Autodesk Inventor part; units mm, degrees
ref_plane "YZ Plane" through (0, 0, 0) normal (1, 0, 0) x (0, 1, 0)
ref_plane "XZ Plane" through (0, 0, 0) normal (0, 1, 0) x (-1, 0, 0)
ref_plane "XY Plane" through (0, 0, 0) normal (0, 0, 1) x (1, 0, 0)
sketch "Sketch1" plane through (0, 0, 0) normal (0, 1, 0) x (-1, 0, 0)
  circle A0 centre (0, 0) radius 20
  dimension "d0" = 40
extrude "Extrusion1" add sketch "Sketch1" along normal blind 26
sketch "Sketch2" plane through (0, 26, 0) normal (0, 1, 0) x (1, 0, 0)
  circle A0 centre (0, 0) radius 19.95
  dimension "d3" = 39.9
extrude "Extrusion2" add sketch "Sketch2" along normal blind 5
sketch "Sketch3" plane through (0, 31, 0) normal (0, 1, 0) x (1, 0, 0)
  circle A0 centre (0, 0) radius 10
  dimension "d6" = 20
extrude "Extrusion3" add sketch "Sketch3" along normal blind 5
sketch "Sketch4" plane through (0, 36, 0) normal (0, 1, 0) x (1, 0, 0)
  circle A0 centre (0, 0) radius 3
  dimension "d9" = 6
extrude "Extrusion4" add sketch "Sketch4" along normal blind 15
sketch "Sketch5" plane through (0, 51, 0) normal (0, 1, 0) x (1, 0, 0)
  circle A0 centre (0, 0) radius 3
  circle A1 centre (0, 0) radius 3
  line L0 (-1.9261, -2.3) -> (1.9261, -2.3)
  dimension "d12" = 2.3
extrude "Extrusion5" cut sketch "Sketch5" against normal blind 10 contours L0 A0 picked at (0.4482, -2.4273)
fillet "Fillet1" radius 2 1 edges at (20, 0, 0)
chamfer "Chamfer1" distance 1 angle 45 2 edges at (-19.95, 31, 0) (-10, 36, 0)
chamfer "Chamfer2" distance 0.5 angle 45 2 edges at (2.7183, 51, 1.2692) (-1.2692, 51, -2.7183)
sketch "Sketch6" plane through (0, 31, 0) normal (0, 1, 0) x (1, 0, 0)
  point P0 (0, 0)
  point P1 (0, 15)
  point P2 (-12.9904, -7.5)
  point P3 (12.9904, -7.5)
  dimension "d23" = 15
  dimension "d26" = 360
hole "Hole1" at (0, 31, -15) at (-12.9904, 31, 7.5) at (12.9904, 31, 7.5) direction (0, -1, 0) diameter 3.4 depth 5 tip angle 118 countersink diameter 3.8 countersink angle 90
properties part number "Encoder" material "Stainless Steel"
Build history of the part. All positions in model axes, mm. A direction names the side the tool comes from. Give positions to 0.01 mm unless a question says otherwise; leave off trailing zeros. Write each loop counter-clockwise with the first axis right and the second up, starting at its lowest first coordinate (ties: lowest second). Pieces come first, ordered by that corner, then holes. Notation, with made-up numbers: (0.5, -6.75) - (22.5, -6.75) arc R25 cw to (22.5, 7.25) - close; hole circle Ø6 at (85, 12.5). An arc over 180 degrees is marked (long way). Use one line per item in the form item = value. Start each with the question number.
1. Band-saw the part on A-A on y = 42.5. Write the cut outline in (x, z).
2. Drop flat-ended pins along their axis: pin 1 Ø8 at (y, z) = (10, -16) entering from +X; pin 2 Ø5.5 at (x, z) = (12.99, 7.5) entering from +Y; pin 3 Ø4 at (x, z) = (-8, 15) entering from -Y; pin 4 Ø4 at (x, y) = (15.5, 17.5) entering from +Z. Give the stop position or say it passes through.
3. 3-axis set-ups, long thin cutter, end or side, ignore diameter. For faces 5 (the face through (0, 46, 2.3)), 6 (the face through (19.03, 27.97, 5.99)): which of +Z, -Z, +X, -X, +Y, -Y reach the whole face in a straight line?
4. Probe line 1 (X direction, y = 27.7, z = 7.5); line 2 (Z direction, x = 0, y = 27); line 3 (X direction, y = 28, z = 7). List the from-to ranges inside material, lowest first. Write a range as [from, to].
5. Band-saw the part on B-B on y = 8. Write the cut outline in (x, z), plus the area to 3 significant figures.
6. Two-plate mould, pull along Z, no slides. Class faces 1 (the face through (0, 51, 0)), 2 (the face through (-2.17, 32.97, -9.76)), 3 (the face through (11.305, 28.366, 7.279)), 4 (the face through (13.239, 25.156, 7.659)): released by +Z, released by -Z, zero draft, split by the parting line, or undercut.
Conclusion:
q1.outline = (-1.93, 2.3) arc R3 ccw (long way) to (1.93, 2.3) - close
q2.pin_1 = 16
q2.pin_2 = 31
q2.pin_3 = 0
q2.pin_4 = 14.76
q3.face_5 = +Z, +X, -X, +Y
q3.face_6 = +Y
q4.line_1 = [-18.49, -14.69], [-11.29, 11.29], [14.69, 18.49]
q4.line_2 = [-19.95, -16.7], [-13.3, 19.95]
q4.line_3 = [-18.68, -14.62], [-11.37, 11.37], [14.62, 18.68]
q5.outline = circle Ø40 at (0, 0)
q5.area = 1,260 mm²
q6.face_1 = zero draft
q6.face_2 = split by the parting line
q6.face_3 = undercut
q6.face_4 = undercut
